from build123d import *

# Parameters (mm, degrees)
F1_DEPTH = 0.75


# Not quite as in the source:
# - a feature names something its author has since deleted; it is built from what else it names


with BuildPart() as f1:
    # F0 (on Right) → F1 (new body, symmetric)
    with BuildSketch(Plane.YZ):
        with BuildLine():
            Line((-22.3, -0.8), (-22.3, 5.0912878854))
            ThreePointArc((-22.3, 5.0912878854), (-28.2361690228, 4.0365729174), (-33.9360169573, 6.0018362214))
            Line((-33.9360169573, 6.0018362214), (-27.9066450894, 2))
            Line((-27.9066450894, 2), (-26.5, 2))
            ThreePointArc((-26.5, 2), (-26.3585786438, 1.9414213562), (-26.3, 1.8))
            Line((-26.3, 1.8), (-26.3, -0.8))
            ThreePointArc((-26.3, -0.8), (-26.2414213562, -0.9414213562), (-26.1, -1))
            Line((-26.1, -1), (-22.5, -1))
            ThreePointArc((-22.5, -1), (-22.3585786438, -0.9414213562), (-22.3, -0.8))
        make_face()
    extrude(amount=F1_DEPTH, both=True)


solid = f1.part
The listing builds one solid part. Answer for the finished solid, in the listing's coordinates (mm). A direction names the side the tool comes from. Give positions to 0.01 mm unless a question says otherwise; leave off trailing zeros. Write each loop counter-clockwise with the first axis right and the second up, starting at its lowest first coordinate (ties: lowest second). Pieces come first, ordered by that corner, then holes. Notation, with made-up numbers: (-8.5, 10) -> (17.5, 10) arc R30 ccw to (17.5, 45) -> close; hole circle Ø1 at (21.25, 36). An arc over 180 degrees is marked (long way). One line per question, with ' | ' between items. Start each with the question number.
1. Section B-B (x = -0.55) is taken. Determine the outline of the cut face in (y, z), plus the area to 3 significant figures.
2. Section D-D (z = 3.5) is taken. Determine the outline of the cut face in (x, y).
3. Section A-A (z = 4.75) is taken. Determine the outline of the cut face in (x, y), plus the area to 3 significant figures.
4. Find the intervals of material crossed by probe 1 along Z at (x, y) = (-0.05, -27.25); probe 2 along Y at (x, z) = (0.5, -0.5); probe 3 along Y at (x, z) = (0.4, 5), in increasing order.
5. Given pin 1 Ø0.8 at (x, z) = (0, 1) entering from -Y, flat-ended and moving along its own axis, determine where the tip first touches the part or whether it passes through.
6. For faces 1 (the flat face through (0, -26.3, 1)), 2 (the flat face through (-0.75, -26, 2)), determine the directions among +Z, -Z, +X, -X, +Y, -Y from which every point of the face is accessible in a straight line to the end or side of a thin tool.
7. Section C-C (y = -29.75) is taken. Determine the outline of the cut face in (x, z), plus the area to 3 significant figures.
Response values:
1) outline: (-33.94, 6) -> (-27.91, 2) -> (-26.5, 2) arc R0.2 cw to (-26.3, 1.8) -> (-26.3, -0.8) arc R0.2 ccw to (-26.1, -1) -> (-22.5, -1) arc R0.2 ccw to (-22.3, -0.8) -> (-22.3, 5.09) arc R12 cw to start | area: 29.3 mm2
2) outline: (-0.75, -30.17) -> (0.75, -30.17) -> (0.75, -22.3) -> (-0.75, -22.3) -> close
3) outline: (-0.75, -32.05) -> (0.75, -32.05) -> (0.75, -31.48) -> (-0.75, -31.48) -> close; (-0.75, -23.12) -> (0.75, -23.12) -> (0.75, -22.3) -> (-0.75, -22.3) -> close | area: 2.10 mm2
4) probe 1: 2 to 4 | probe 2: -26.3 to -22.3 | probe 3: -32.43 to -32.1, -22.5 to -22.3
5) pin 1: y = -26.3
6) face 1: -Z, +X, -X, -Y | face 2: +Z, -Z, -X, +Y, -Y
7) outline: (-0.75, 3.22) -> (0.75, 3.22) -> (0.75, 4.25) -> (-0.75, 4.25) -> close | area: 1.54 mm2
